from build123d import *

# Parameters (mm, degrees)
P_IDAT_VYSUNUT_M1_DEPTH  = 50
SKICA7_W                 = 50
SKICA7_H                 = 164
P_IDAT_VYSUNUT_M5_DEPTH  = 30
P_IDAT_VYSUNUT_M16_DEPTH = 5
LINPOLE1_COUNT           = 4
LINPOLE1_PITCH           = 53
P_IDAT_VYSUNUT_M17_DEPTH = 55
LINPOLE2_COUNT           = 3
LINPOLE2_PITCH           = 55
P_IDAT_VYSUNUT_M18_DEPTH = 110
P_IDAT_VYSUNUT_M19_DEPTH = 20
SKICA29_R                = 2.5
ODEBRAT_VYSUNUT_M1_DEPTH = 387.276474167


with BuildPart() as part:
    # Skica1 → Přidat vysunutím1 (new body)
    with BuildSketch(Plane.XY):
        Polygon((0, 0), (200, 0), (200, 350), (70, 220), (0, 220), align=None)
    extrude(amount=P_IDAT_VYSUNUT_M1_DEPTH)

    # Skica7 → Přidat vysunutím5 (add)
    with BuildSketch(Plane.XY.offset(50)):
        with Locations((175, 132)):
            Rectangle(SKICA7_W, SKICA7_H)
    extrude(amount=P_IDAT_VYSUNUT_M5_DEPTH)

    # Skica23 → Přidat vysunutím16 (add)
    with BuildSketch(Plane.XZ.offset(-50)):
        with BuildLine():
            Line((200, 80), (237.75041097, 66.774778957))
            Line((237.75041097, 66.774778957), (259.241395164, 128.119196783))
            Line((259.241395164, 128.119196783), (240.366189679, 134.731807304))
            ThreePointArc((240.366189679, 134.731807304), (203.062547088, 161.906480142), (186.977305802, 205.164885189))
            Line((186.977305802, 205.164885189), (185.40091467, 230))
            Line((185.40091467, 230), (105.40091467, 230))
            Line((105.40091467, 230), (150, 100))
            Line((150, 100), (150, 80))
            Line((150, 80), (200, 80))
        make_face()
    p_idat_vysunut_m16 = extrude(amount=-P_IDAT_VYSUNUT_M16_DEPTH)

    # LinPole1: Přidat vysunutím16 ×4
    with Locations(*[(0, i * LINPOLE1_PITCH, 0) for i in range(1, LINPOLE1_COUNT)]):
        add(p_idat_vysunut_m16)

    # Skica26 → Přidat vysunutím17 (add)
    with BuildSketch(Plane.XZ.offset(-50)):
        with BuildLine():
            Line((140.606634732, 127.380325757), (105.40091467, 230))
            Line((105.40091467, 230), (110.686974043, 230))
            Line((110.686974043, 230), (144.970270535, 130.069059465))
            ThreePointArc((144.970270535, 130.069059465), (188.679692745, 95.127098247), (239.4035636, 71.493580328))
            Line((239.4035636, 71.493580328), (237.75041097, 66.774778957))
            ThreePointArc((237.75041097, 66.774778957), (185.516396292, 91.207581344), (140.606634732, 127.380325757))
        make_face()
        with BuildLine():
            Line((185.40091467, 230), (185.40091467, 202.92837758))
            ThreePointArc((185.40091467, 202.92837758), (211.446760209, 154.790204461), (259.241395164, 128.119196783))
            Line((259.241395164, 128.119196783), (257.588242534, 123.400395411))
            ThreePointArc((257.588242534, 123.400395411), (207.477117523, 151.738564679), (180.40091467, 202.542658277))
            Line((180.40091467, 202.542658277), (180.40091467, 230))
            Line((180.40091467, 230), (185.40091467, 230))
        make_face()
    p_idat_vysunut_m17 = extrude(amount=-P_IDAT_VYSUNUT_M17_DEPTH)

    # LinPole2: Přidat vysunutím17 ×3
    with Locations(*[(0, i * LINPOLE2_PITCH, 0) for i in range(1, LINPOLE2_COUNT)]):
        add(p_idat_vysunut_m17)

    # Skica27 → Přidat vysunutím18 (add)
    with BuildSketch(Plane.XY.offset(50)):
        Polygon((53.405814175, 139.046612135), (87.877814115, 167.972054571), (68.594185825, 190.953387865), (34.122185885, 162.027945429), align=None)
    extrude(amount=P_IDAT_VYSUNUT_M18_DEPTH)

    # Skica28 → Přidat vysunutím19 (add)
    with BuildSketch(Plane.XY.offset(160)):
        Polygon((55.18840807, 179.704604695), (74.472036361, 156.723271402), (87.877814115, 167.972054571), (68.594185825, 190.953387865), align=None)
        Polygon((47.527963639, 173.276728598), (66.81159193, 150.295395305), (53.405814175, 139.046612135), (34.122185885, 162.027945429), align=None)
    extrude(amount=P_IDAT_VYSUNUT_M19_DEPTH)

    # Skica29 → Odebrat vysunutím1 (cut, through all)
    with BuildSketch(Plane(origin=(99.806909072, 83.747940591, 0), x_dir=(0, 0, 1), z_dir=(-0.7660444431189739, -0.6427876096865444, 0))):
        with Locations(Location((170, 87.187288924, 0), (0, 0, 270))):
            Circle(SKICA29_R)
    extrude(amount=-ODEBRAT_VYSUNUT_M1_DEPTH, mode=Mode.SUBTRACT)


solid = part.part
Input: part model. Units: mm. Frame: model coordinates. A direction names the side the tool comes from. Coordinates: 2 decimals unless noted, no trailing zeros. Loops run counter-clockwise (first coordinate to the right, second up) from the corner with the lowest first, then second, coordinate; pieces in that order, holes last. Notation, with made-up numbers: (40, 29) -> (66, 29) arc R29 ccw to (66, 50) -> close; hole circle Ø8 at (-20.5, -13). An arc over 180 degrees is marked (long way). Write item = value, one per line. Start each with the question number.
Item 1: First-contact query: P1, Ø2.5, axis at x = 188, z = 209.5, coming from the -Y side; P2, Ø22, axis at y = 77, z = 215.5, coming from the -X side; P3, Ø6, axis at x = 81.5, z = 150, coming from the +Y side; P4, Ø8, axis at x = 60.5, y = 160, coming from the +Z side. Flat tips, straight axial feed; report the tip coordinate or a pass-through.
Item 2: Cut plane A-A, the plane y = 90. Return loops of the section in (x, z), plus the area to 3 significant figures.
Item 3: Material intervals for line 1 (Y direction, x = 180.5, z = 116); line 2 (Z direction, x = 174, y = 271); line 3 (Z direction, x = 164.5, y = 145), sorted ascending.
Item 4: Mould query, pull axis Y, two halves, no side actions, for faces 1 (the face through (78.37, 179.3, 114.09)), 2 (the face through (208.05, 78.664, 151.156)), 3 (the face through (214.202, 105.465, 75.025)). Classes: pulls with the +Y half, pulls with the -Y half, needs draft (parallel to the pull), parting line crosses it, or undercut.
Item 5: Cut plane D-D, the plane y = 317. Return loops of the section in (x, z), plus the area to 3 significant figures.
Item 6: Cut plane B-B, the plane z = 30. Return loops of the section in (x, y).
Item 7: Reachability of faces 4 (the face through (214.202, 52.465, 75.025)), 5 (the face through (208.05, 184.664, 151.156)), 6 (the face through (210.9, 131.34, 155.35)), 7 (the face through (183, 214, 152)) from +Z, -Z, +X, -X, +Y, -Y: full face, straight path, thin tool, end or side. Return the list, or none.
Ans:
q1.P1 = through
q1.P2 = 106.6
q1.P3 = 179.15
q1.P4 = 180
q2.outline = (0, 0) -> (200, 0) -> (200, 80) -> (150, 80) -> (150, 50) -> (0, 50) -> close; (105.4, 230) -> (140.61, 127.38) arc R240.32 ccw to (237.75, 66.77) -> (239.4, 71.49) arc R235.32 cw to (144.97, 130.07) -> (110.69, 230) -> close; (180.4, 202.54) arc R103 ccw to (257.59, 123.4) -> (259.24, 128.12) arc R98.03 cw to (185.4, 202.93) -> (185.4, 230) -> (180.4, 230) -> close
q2.area = 13,300 mm²
q3.line_1 = 50 to 55, 103 to 108, 156 to 161, 209 to 214
q3.line_2 = 0 to 50
q3.line_3 = 0 to 80, 105.93 to 112.33
q4.face_1 = pulls with the +Y half
q4.face_2 = undercut
q4.face_3 = needs draft
q5.outline = (167, 0) -> (200, 0) -> (200, 50) -> (167, 50) -> close
q5.area = 1,650 mm²
q6.outline = (0, 0) -> (200, 0) -> (200, 350) -> (70, 220) -> (0, 220) -> close
q7.face_4 = -Z, +Y, -Y
q7.face_5 = none
q7.face_6 = +Z, +X
q7.face_7 = +Y
